```python
from build123d import *

# Parameters (mm, degrees)
PAD_DEPTH             = 1.6
POLARPATTERN_COUNT    = 4
POCKET_DEPTH          = 5
POLARPATTERN001_COUNT = 4
FILLET_R              = 12


with BuildPart() as part:
    # Sketch → Pad (new body)
    with BuildSketch(Plane.XY):
        with BuildLine():
            Line((0, 0), (-85, 0))
            ThreePointArc((-73.070068, 43.425398), (-81.963272, 22.517151), (-85, 0))
            ThreePointArc((0, 85), (-42.034755, 73.878816), (-73.070068, 43.425398))
            Line((0, 0), (0, 85))
        make_face()
    pad = extrude(amount=PAD_DEPTH)

    # PolarPattern: Pad ×4 about axis
    polarpattern_axis = Axis((0, 0, 0), (0, 0, 1))
    for i in range(1, POLARPATTERN_COUNT):
        add(pad.rotate(polarpattern_axis, i * 360 / POLARPATTERN_COUNT))

    # Sketch001 → Pocket (cut)
    with BuildSketch(Plane.XY):
        with BuildLine():
            ThreePointArc((-91.627857, -50.5), (-75, 0), (-91.627857, 50.5))
            Line((-91.627857, 50.5), (-91.627857, -50.5))
        make_face()
    pocket = extrude(amount=POCKET_DEPTH, mode=Mode.SUBTRACT)

    # PolarPattern001: Pocket ×4 about axis
    polarpattern001_axis = Axis((0, 0, 0), (0, 0, 1))
    for i in range(1, POLARPATTERN001_COUNT):
        add(pocket.rotate(polarpattern001_axis, i * 360 / POLARPATTERN001_COUNT), mode=Mode.SUBTRACT)

    # Fillet
    fillet_edges = [part.edges().sort_by_distance(p)[0] for p in [
        (-80, 28.722813, 0.8),
        (-80, -28.722813, 0.8),
        (-28.722813, 80, 0.8),
        (28.722813, 80, 0.8),
        (80, 28.722813, 0.8),
        (80, -28.722813, 0.8),
        (-28.722813, -80, 0.8),
        (28.722813, -80, 0.8),
    ]]
    fillet(fillet_edges, radius=FILLET_R)


solid = part.part
```
Geometry check sheet. Reference: the model listing, model coordinates, mm. Round coordinates to 2 decimals unless told otherwise and drop trailing zeros. Loops run counter-clockwise (first coordinate to the right, second up) from the corner with the lowest first, then second, coordinate; pieces in that order, holes last. Notation, with made-up numbers: (84, 77) -> (123, 77) arc R25 ccw to (123, 91) -> close; hole circle Ø1 at (5.25, -12.75). An arc over 180 degrees is marked (long way). Use a Markdown table: item, result.
(1) Mould release check, pull along Y, two halves, no side actions. Record for faces 1 (the cylindrical face through (0, -75, 1)), 2 (the cylindrical face through (0, 75, 1)), 3 (the cylindrical face through (75, 0, 1)): released by +Y, released by -Y, zero draft, split by the parting line, or undercut.
Calculated:
| item | result |
|---|---|
| face 1 | released by -Y |
| face 2 | released by +Y |
| face 3 | undercut |
(2) Scan lines: probe 1 along X at (y, z) = (-28, 0.95); probe 2 along Y at (x, z) = (40, 0.95); probe 3 along X at (y, z) = (-11.5, 0.4). Record each from-to range of solid material in increasing order.
Calculated:
| item | result |
|---|---|
| probe 1 | -79.24 to 79.24 |
| probe 2 | -75 to 75 |
| probe 3 | -75.78 to 75.78 |
(3) Sectioned sample at B-B (x = -57.5). Enter the section's corners in (y, z).
Calculated:
| item | result |
|---|---|
| outline | (-62.6, 0) -> (62.6, 0) -> (62.6, 1.6) -> (-62.6, 1.6) -> close |
(4) Sectioned sample at A-A (y = -51.5). Enter the section's corners in (x, z).
Calculated:
| item | result |
|---|---|
| outline | (-67.62, 0) -> (67.62, 0) -> (67.62, 1.6) -> (-67.62, 1.6) -> close |
